Source: CAD feature listing. Evaluate the final solid. Frame: model axes, mm. A direction names the side the tool comes from. Give positions to 0.01 mm unless a question says otherwise; leave off trailing zeros. Order: outer loops, then holes, each group sorted by start corner. A loop starts at its lowest first (then second) coordinate and runs counter-clockwise, first axis right, second up. Notation, with made-up numbers: M 14.5,79.25 L 64.5,79.25 A24 cw 64.5,101.25 Z; hole C 12,70 d8. An arc over 180 degrees is marked long. Use CSV: the item, a comma, the result in double quotes. Start each with the question number.
1. Section query D-D, the plane z = 2.25. Return the cut outline in (x, y).
2. Line query: line 1 along X through (y, z) = (4, -1.45); line 2 along X through (y, z) = (2, -1.8); line 3 along Z through (x, y) = (-5.25, 4.25). Output: solid intervals per line, ascending. Write a range as [from, to].
3. Section query A-A, the plane y = 5.5. Return the cut outline in (x, z), plus the area to 3 significant figures.
4. Mould query, pull axis Z, two halves, no side actions, for faces 3 (the flat face through (0, 5, 2.95)), 4 (the flat face through (0, 9, 0)), 5 (the flat face through (5.55, 4, 0)), 6 (the flat face through (-6.05, 5, 0)). Classes: released by +Z, released by -Z, zero draft, split by the parting line, or undercut.
5. Section query C-C, the plane z = -0.35. Return the cut outline in (x, y).
6. Pin query (flat end, axial travel): P1, Ø1, axis at x = 3, z = 1.5, coming from the -Y side; P2, Ø2, axis at x = -3, z = 2.5, coming from the -Y side. Return the tip coordinate at first contact, or that it passes through.
7. Reachability of faces 1 (the flat face through (-5.446, 10.507, 0.041)), 2 (the flat face through (-4, 4, 2.45)) from +Z, -Z, +X, -X, +Y, -Y: full face, straight path, thin tool, end or side. Return the list, or none.
8. Section query B-B, the plane x = 0. Return the cut outline in (y, z), plus the area to 3 significant figures.
from build123d import *
from OCP.BRepFilletAPI import BRepFilletAPI_MakeChamfer

# Parameters (mm, degrees)
SKETCH1_W           = 12.1
SKETCH1_H           = 5.9
BOSS_EXTRUDE1_DEPTH = 11
CHAMFER1_SIZE       = 1
CHAMFER1_SIZE2      = 1.191753593
CUT_EXTRUDE3_DEPTH  = 14.871283286
CUT_EXTRUDE4_DEPTH  = 9


with BuildPart() as part:
    # Sketch1 → Boss-Extrude1 (new body)
    with BuildSketch(Plane(origin=(0, 0, 0), x_dir=(1, 0, 0), z_dir=(0, 1, 0))):
        Rectangle(SKETCH1_W, SKETCH1_H)
    extrude(amount=BOSS_EXTRUDE1_DEPTH)

    # Chamfer1: one chamfer whose edges measure the first distance from different faces: ONE call of the kernel's chamfer builder (chamfer() names one face for all edges)
    chamfer1_edges_1 = [part.edges().sort_by_distance(p)[0] for p in [
        (6.05, 11, 0),
    ]]
    chamfer1_side_1 = [part.faces().sort_by_distance(p)[0] for p in [
        (6.05, 5.5, 0),
    ]]
    chamfer1_edges_2 = [part.edges().sort_by_distance(p)[0] for p in [
        (0, 11, -2.95),
    ]]
    chamfer1_side_2 = [part.faces().sort_by_distance(p)[0] for p in [
        (0, 5.5, -2.95),
    ]]
    chamfer1_edges_3 = [part.edges().sort_by_distance(p)[0] for p in [
        (-6.05, 11, 0),
    ]]
    chamfer1_side_3 = [part.faces().sort_by_distance(p)[0] for p in [
        (-6.05, 5.5, 0),
    ]]
    chamfer1_edges_4 = [part.edges().sort_by_distance(p)[0] for p in [
        (0, 11, 2.95),
    ]]
    chamfer1_side_4 = [part.faces().sort_by_distance(p)[0] for p in [
        (0, 5.5, 2.95),
    ]]
    chamfer1 = BRepFilletAPI_MakeChamfer(part.part.solid().wrapped)
    for e in chamfer1_edges_1:
        chamfer1.Add(CHAMFER1_SIZE, CHAMFER1_SIZE2, e.wrapped, chamfer1_side_1[0].wrapped)  # the first distance lies on this face
    for e in chamfer1_edges_2:
        chamfer1.Add(CHAMFER1_SIZE, CHAMFER1_SIZE2, e.wrapped, chamfer1_side_2[0].wrapped)  # the first distance lies on this face
    for e in chamfer1_edges_3:
        chamfer1.Add(CHAMFER1_SIZE, CHAMFER1_SIZE2, e.wrapped, chamfer1_side_3[0].wrapped)  # the first distance lies on this face
    for e in chamfer1_edges_4:
        chamfer1.Add(CHAMFER1_SIZE, CHAMFER1_SIZE2, e.wrapped, chamfer1_side_4[0].wrapped)  # the first distance lies on this face
    add(Compound.cast(chamfer1.Shape()), mode=Mode.REPLACE)

    # Sketch6 → Cut-Extrude3 (cut, through all)
    with BuildSketch(Plane.XY.offset(2.95)):
        with BuildLine():
            Line((-4.858246407, 11), (4.858246407, 11))
            ThreePointArc((4.858246407, 11), (0, 10.85), (-4.858246407, 11))
        make_face()
    extrude(amount=-CUT_EXTRUDE3_DEPTH, mode=Mode.SUBTRACT)

    # Sketch7 → Cut-Extrude4 (cut)
    with BuildSketch(Plane.XZ):
        Polygon((-2.05, -1), (-2.05, -2.45), (-5.55, -2.45), (-5.55, 2.45), (-2.05, 2.45), (-2.05, 1), (-1.65, 1), (-1.65, 1.65), (1.65, 1.65), (1.65, 1), (2.05, 1), (2.05, 2.45), (5.55, 2.45), (5.55, -2.45), (2.05, -2.45), (2.05, -1), (1.65, -1), (1.65, -1.65), (-1.65, -1.65), (-1.65, -1), align=None)
    extrude(amount=-CUT_EXTRUDE4_DEPTH, mode=Mode.SUBTRACT)


solid = part.part
Result set:
1,outline,"M -6.05,0 L -5.55,0 L -5.55,9 L -2.05,9 L -2.05,0 L 2.05,0 L 2.05,9 L 5.55,9 L 5.55,0 L 6.05,0 L 6.05,10 L 5.35,10.59 L -5.35,10.59 L -6.05,10 Z"
2,line 1,"[-6.05, -5.55], [-2.05, -1.65], [1.65, 2.05], [5.55, 6.05]"
2,line 2,"[-6.05, -5.55], [-2.05, 2.05], [5.55, 6.05]"
2,line 3,"[-2.95, -2.45], [2.45, 2.95]"
3,outline,"M -6.05,-2.95 L 6.05,-2.95 L 6.05,2.95 L -6.05,2.95 Z; hole M -5.55,-2.45 L -2.05,-2.45 L -2.05,-1 L -1.65,-1 L -1.65,-1.65 L 1.65,-1.65 L 1.65,-1 L 2.05,-1 L 2.05,-2.45 L 5.55,-2.45 L 5.55,2.45 L 2.05,2.45 L 2.05,1 L 1.65,1 L 1.65,1.65 L -1.65,1.65 L -1.65,1 L -2.05,1 L -2.05,2.45 L -5.55,2.45 Z"
3,area,"24.6 mm2"
4,face 3,"released by +Z"
4,face 4,"undercut"
4,face 5,"undercut"
4,face 6,"zero draft"
5,outline,"M -6.05,0 L -5.55,0 L -5.55,9 L 5.55,9 L 5.55,0 L 6.05,0 L 6.05,10 L 4.86,11 A78.75 cw -4.86,11 L -6.05,10 Z"
6,P1,"y = 9"
6,P2,"y = 0"
7,face 1,"+Z, -Z, -X, +Y"
7,face 2,"-Y"
8,outline,"M 0,-2.95 L 10,-2.95 L 10.85,-1.94 L 10.85,1.94 L 10,2.95 L 0,2.95 L 0,1.65 L 9,1.65 L 9,-1.65 L 0,-1.65 Z"
8,area,"33.5 mm2"
